Source: CAD feature listing. Evaluate the final solid. Frame: model axes, mm. A direction names the side the tool comes from. Coordinates: 2 decimals unless noted, no trailing zeros. Order: outer loops, then holes, each group sorted by start corner. A loop starts at its lowest first (then second) coordinate and runs counter-clockwise, first axis right, second up.
```python
from build123d import *

# Parameters (mm, degrees)
F1_DEPTH = 1.5
F4_W     = 60
F4_H     = 110
F5_DEPTH = 3
F6_R     = 5
F7_R     = 5


# Not quite as in the source:
# - a feature names something its author has since deleted; it is built from what else it names


with BuildPart() as f1:
    # F0 (on Top) → F1 (new body, symmetric)
    with BuildSketch(Plane.XY):
        with BuildLine():
            Line((31.2800427974, 63.3035998776), (0, 63.3035998776))
            Line((0, 63.3035998776), (0, 0))
            Line((0, 0), (64, 0))
            Line((64, 0), (64, 52.0472386562))
            ThreePointArc((64, 52.0472386562), (63.9147152873, 52.211069065), (63.7315959713, 52.2351771803))
            Line((63.7315959713, 52.2351771803), (62.4040530693, 51.7519910793))
            Line((62.4040530693, 51.7519910793), (60.2493261663, 57.6720545902))
            ThreePointArc((60.2493261663, 57.6720545902), (59.9996605802, 57.9445167667), (60.3688606618, 57.9283971431))
            Line((60.3688606618, 57.9283971431), (62.8120614758, 58.8176495157))
            ThreePointArc((62.8120614758, 58.8176495157), (63.0845236523, 59.0673151018), (63.0684040287, 58.6981150202))
            Line((63.0684040287, 58.6981150202), (63.2443290661, 58.2147649522))
            ThreePointArc((63.2443290661, 58.2147649522), (63.3805037813, 58.0899838157), (63.5608251122, 58.1299600923))
            Line((63.5608251122, 58.1299600923), (63.9285575219, 58.4385242216))
            ThreePointArc((63.9285575219, 58.4385242216), (63.9812615574, 58.5072094579), (64, 58.5917331103))
            Line((64, 58.5917331103), (64, 69.8918015034))
            Line((64, 69.8918015034), (32.9901435141, 58.6051367736))
            Line((32.9901435141, 58.6051367736), (32.7849314281, 59.1689523461))
            Line((32.7849314281, 59.1689523461), (64, 73.3944786626))
            Line((64, 73.3944786626), (63.4156380227, 75))
            Line((63.4156380227, 75), (59.0299314225, 75))
            Line((59.0299314225, 75), (57.3566676351, 74.3909817873))
            Line((57.3566676351, 74.3909817873), (57.8012938214, 73.1693813803))
            ThreePointArc((57.8012938214, 73.1693813803), (58.0509594075, 72.8969192038), (57.681759326, 72.9130388275))
            Line((57.681759326, 72.9130388275), (31.2800427974, 63.3035998776))
        make_face()
    extrude(amount=F1_DEPTH, both=True)

    # F2: F1 across face


with BuildPart() as f1_1:
    add(f1.part)
    add(f1.part.mirror(Plane(origin=(0, 31.6517999388, 0), x_dir=(0, -1, 0), z_dir=(-1, 0, 0))))

    # F3: F1 across face


with BuildPart() as f1_2:
    add(f1_1.part)
    add(f1_1.part.mirror(Plane.XZ))

    # F4 (on face) → F5 (cut, through all)
    with BuildSketch(Plane(origin=(0, 0, -1.5), x_dir=(1, 0, 0), z_dir=(0, 0, -1))):
        Rectangle(F4_W, F4_H)
    extrude(amount=-F5_DEPTH, mode=Mode.SUBTRACT)

    # F6
    f6_edges = [f1_2.edges().sort_by_distance(p)[0] for p in [
        (-64, -69.891802, 0),
        (64, -69.891802, 0),
        (64, 69.891802, 0),
        (-64, 69.891802, 0),
    ]]
    fillet(f6_edges, radius=F6_R)

    # F7
    f7_edges = [f1_2.edges().sort_by_distance(p)[0] for p in [
        (-30, 55, 0),
        (-30, -55, 0),
        (30, -55, 0),
        (30, 55, 0),
    ]]
    fillet(f7_edges, radius=F7_R)


solid = f1_2.part
```
Q1. Section query A-A on y = 38.5. Output: boundary loops of the cut face in (x, z).
Solutions:
outline: (-64, -1.5) - (-30, -1.5) - (-30, 1.5) - (-64, 1.5) - close; (30, -1.5) - (64, -1.5) - (64, 1.5) - (30, 1.5) - close
Q2. Pull-direction query (X, two-part tool) for faces 4 (the flat face through (64, -61, 0)), 5 (the flat face through (61, -75, 0)), 6 (the flat face through (45.31, -63.09, 0.02)); classes: pulls with the +X half, pulls with the -X half, needs draft (parallel to the pull), parting line crosses it, or undercut.
Solutions:
face 4: pulls with the +X half
face 5: needs draft
face 6: undercut
Q3. Section query B-B on x = -1.5. Output: boundary loops of the cut face in (y, z).
Solutions:
outline: (-63.3, -1.5) - (-55, -1.5) - (-55, 1.5) - (-63.3, 1.5) - close; (55, -1.5) - (63.3, -1.5) - (63.3, 1.5) - (55, 1.5) - close
Q4. Set-up query: faces 1 (the flat face through (44, -1, -1.5)), 2 (the flat face through (30, 1, 0)), 3 (the flat face through (0, 63.304, 0)). Return all of +Z, -Z, +X, -X, +Y, -Y with unobstructed straight access to the full face (end or side cutting, diameter ignored); none if empty.
Solutions:
face 1: -Z, +X, -X, +Y, -Y
face 2: +Z, -Z
face 3: +Z, -Z, +Y
Q5. Section query C-C on x = -44.5. Output: boundary loops of the cut face in (y, z).
Solutions:
outline: (-68.12, -1.5) - (-64.51, -1.5) - (-64.51, 1.5) - (-68.12, 1.5) - close; (-62.79, -1.5) - (62.79, -1.5) - (62.79, 1.5) - (-62.79, 1.5) - close; (64.51, -1.5) - (68.12, -1.5) - (68.12, 1.5) - (64.51, 1.5) - close
Q6. Pin query (flat end, axial travel): P1, Ø1.5, axis at x = 4, z = 0.5, coming from the +Y side; P2, Ø0.9, axis at x = 3, z = 0, coming from the -Y side. Return the tip coordinate at first contact, or that it passes through.
Solutions:
P1: stops at y = 63.3
P2: stops at y = -63.3
Q7. Material intervals for line 1 along Y through (x, z) = (-19, -1.05); line 2 along X through (y, z) = (-8.5, -0.75); line 3 along Y through (x, z) = (41, -1.1), sorted ascending.
Solutions:
line 1: y = -63.3 to -55, 55 to 63.3
line 2: x = -64 to -30, 30 to 64
line 3: y = -66.84 to -62.91, -61.52 to 61.52, 62.91 to 66.84
